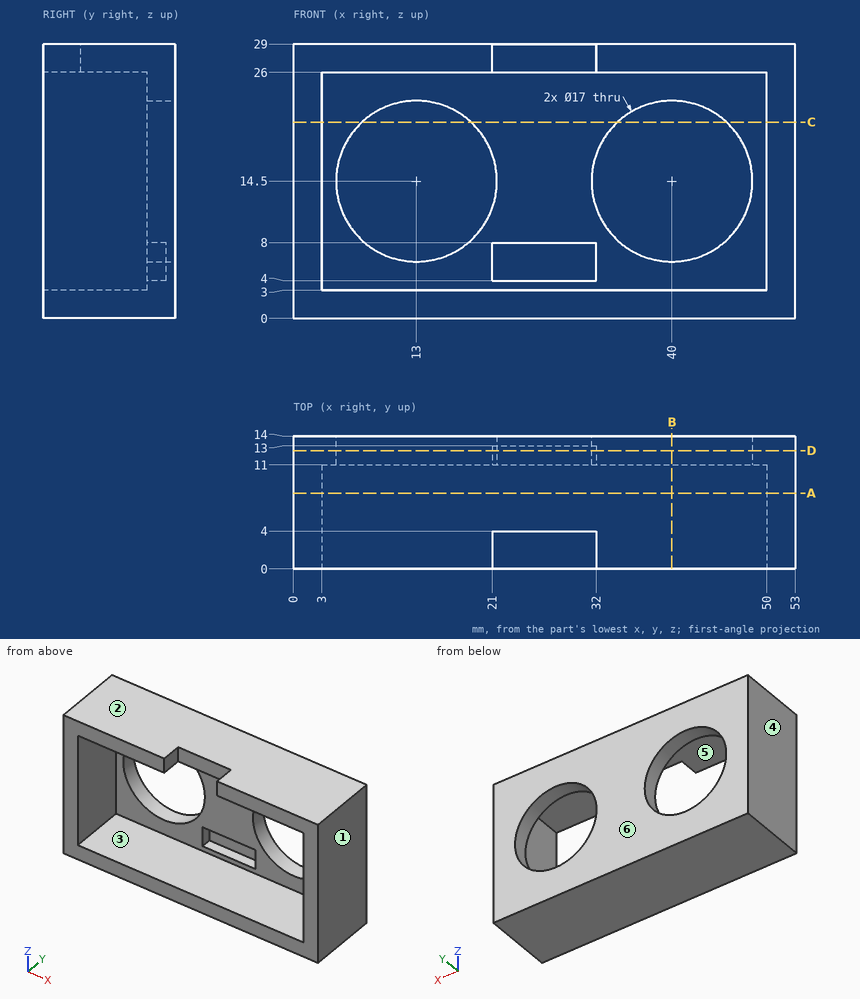
Part print with two shaded views. Sizes in mm from the minimum x, y, z corner. A direction names the side the tool comes from. Round coordinates to 2 decimals unless told otherwise and drop trailing zeros. Order: outer loops, then holes, each group sorted by start corner. A loop starts at its lowest first (then second) coordinate and runs counter-clockwise, first axis right, second up. Notation, with made-up numbers: (14.25, 12.5) - (23.25, 12.5) arc R28 ccw to (23.25, 41.5) - close; hole circle Ø7 at (86, 70.5). An arc over 180 degrees is marked (long way). Answer in a Markdown table with one row per item. Add a question column.
(1) Probe L1, parallel to Z at x = 13, y = 12.05; L2, parallel to Z at x = 34, y = 0.5; L3, parallel to X at y = 9, z = 18. List the from-to ranges inside material, lowest first. Write a range as [from, to].
(2) 3-axis set-ups, long thin cutter, end or side, ignore diameter. For the marked faces 5 and 6: which of +Z, -Z, +X, -X, +Y, -Y reach the whole face in a straight line?
(3) Band-saw the part on C-C on z = 20.75. List the corners of the cut face in (x, y).
(4) Mould opens along X. For the marked faces 1, 2, 3 and 4 say: +X half, -X half, draft (parallel to the pull), parting line (faces both ways), or undercut.
(5) Band-saw the part on D-D on y = 12.5. List the corners of the cut face in (x, z).
(6) Band-saw the part on A-A on y = 8. List the corners of the cut face in (x, z).
(7) Band-saw the part on B-B on x = 40. List the corners of the cut face in (y, z).
(8) Drop flat-ended pins along their axis: pin 1 Ø1.5 at (x, z) = (24, 27.5) entering from -Y; pin 2 Ø2 at (x, z) = (28, 5.5) entering from -Y; pin 3 Ø15.5 at (x, z) = (13, 14.5) entering from -Y. Give the stop position or say it passes through.
Data:
| question | item | result |
|---|---|---|
| 1 | L1 | z = [0, 6], [23, 29] |
| 1 | L2 | z = [0, 3], [26, 29] |
| 1 | L3 | x = [0, 3], [50, 53] |
| 2 | face 5 | -Y |
| 2 | face 6 | +Z, -Z, +X, -X, +Y |
| 3 | outline | (0, 0) - (3, 0) - (3, 11) - (7.24, 11) - (7.24, 14) - (0, 14) - close; (18.76, 11) - (34.24, 11) - (34.24, 14) - (18.76, 14) - close; (45.76, 11) - (50, 11) - (50, 0) - (53, 0) - (53, 14) - (45.76, 14) - close |
| 4 | face 1 | +X half |
| 4 | face 2 | draft |
| 4 | face 3 | undercut |
| 4 | face 4 | -X half |
| 5 | outline | (0, 0) - (53, 0) - (53, 29) - (0, 29) - close; hole circle Ø17 at (13, 14.5); hole (21, 4) - (32, 4) - (32, 8) - (21, 8) - close; hole circle Ø17 at (40, 14.5) |
| 6 | outline | (0, 0) - (53, 0) - (53, 29) - (0, 29) - close; hole (3, 3) - (50, 3) - (50, 26) - (3, 26) - close |
| 7 | outline | (0, 0) - (14, 0) - (14, 6) - (11, 6) - (11, 3) - (0, 3) - close; (0, 26) - (11, 26) - (11, 23) - (14, 23) - (14, 29) - (0, 29) - close |
| 8 | pin 1 | stops at y = 4 |
| 8 | pin 2 | stops at y = 13 |
| 8 | pin 3 | passes through |
